Could you check a few things on this drawing? It's one solid part, dimensions in mm from its lowest x, y, z. Coordinates: 2 decimals unless noted, no trailing zeros. Write each loop counter-clockwise with the first axis right and the second up, starting at its lowest first coordinate (ties: lowest second). Pieces come first, ordered by that corner, then holes. Notation, with made-up numbers: (45.25, -23) - (67.25, -23) arc R23 ccw to (67.25, -5) - close; hole circle Ø6 at (-19, 88). An arc over 180 degrees is marked (long way). Write item = value, one per line. Start each with the question number.
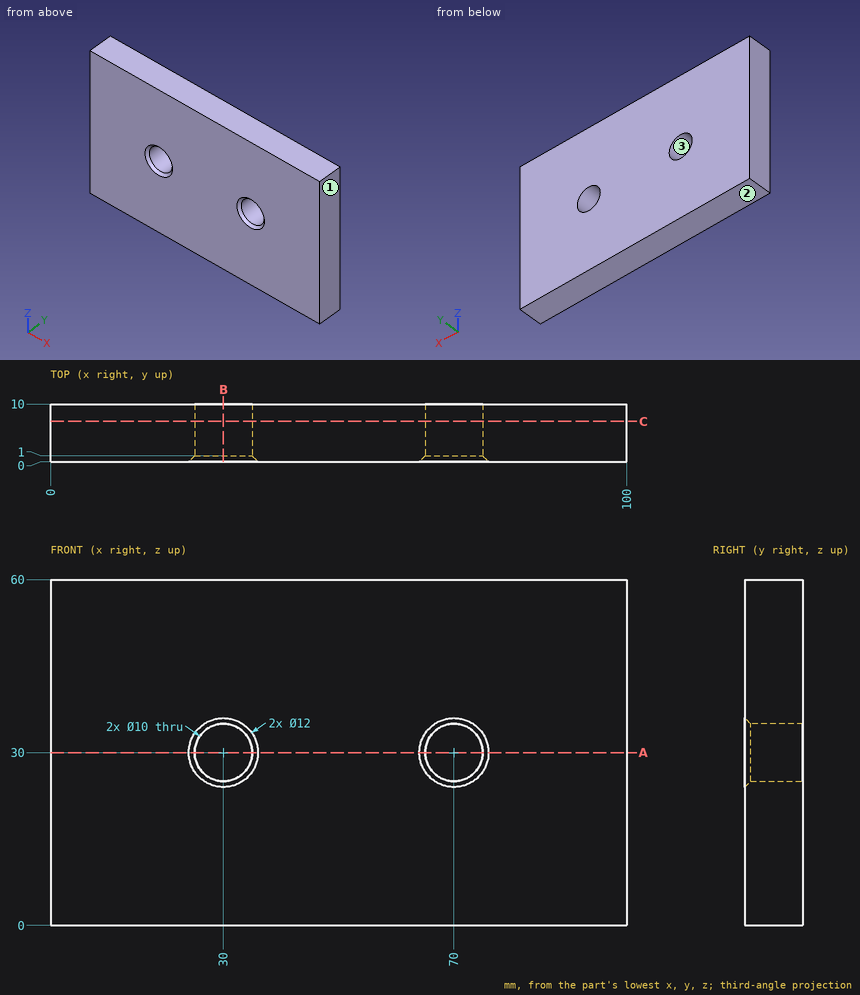
1) Thinking about a two-plate mould opening in X: for the marked faces 1, 2 and 3, which applies, +X half, -X half, draft (parallel to the pull), parting line (faces both ways), or undercut?
2) If I drill on probe 1 along X at (y, z) = (7.5, 30); probe 2 along X at (y, z) = (4.5, 29); probe 3 along Z at (x, y) = (30, 5), over which ranges is the centre line in solid material (lowest first)? Write a range as [from, to].
3) Suppose I cut it at C-C on y = 7. Please give me the cut outline in (x, z).
4) Suppose I cut it at A-A on z = 30. Please give me the cut outline in (x, y).
5) Suppose I cut it at B-B on x = 30. Please give me the cut outline in (y, z).
Reply:
q1.face_1 = +X half
q1.face_2 = draft
q1.face_3 = undercut
q2.probe_1 = [0, 25], [35, 65], [75, 100]
q2.probe_2 = [0, 25.1], [34.9, 65.1], [74.9, 100]
q2.probe_3 = [0, 25], [35, 60]
q3.outline = (0, 0) - (100, 0) - (100, 60) - (0, 60) - close; hole circle Ø10 at (30, 30); hole circle Ø10 at (70, 30)
q4.outline = (0, 0) - (24, 0) - (25, 1) - (25, 10) - (0, 10) - close; (35, 1) - (36, 0) - (64, 0) - (65, 1) - (65, 10) - (35, 10) - close; (75, 1) - (76, 0) - (100, 0) - (100, 10) - (75, 10) - close
q5.outline = (0, 0) - (10, 0) - (10, 25) - (1, 25) - (0, 24) - close; (0, 36) - (1, 35) - (10, 35) - (10, 60) - (0, 60) - close
